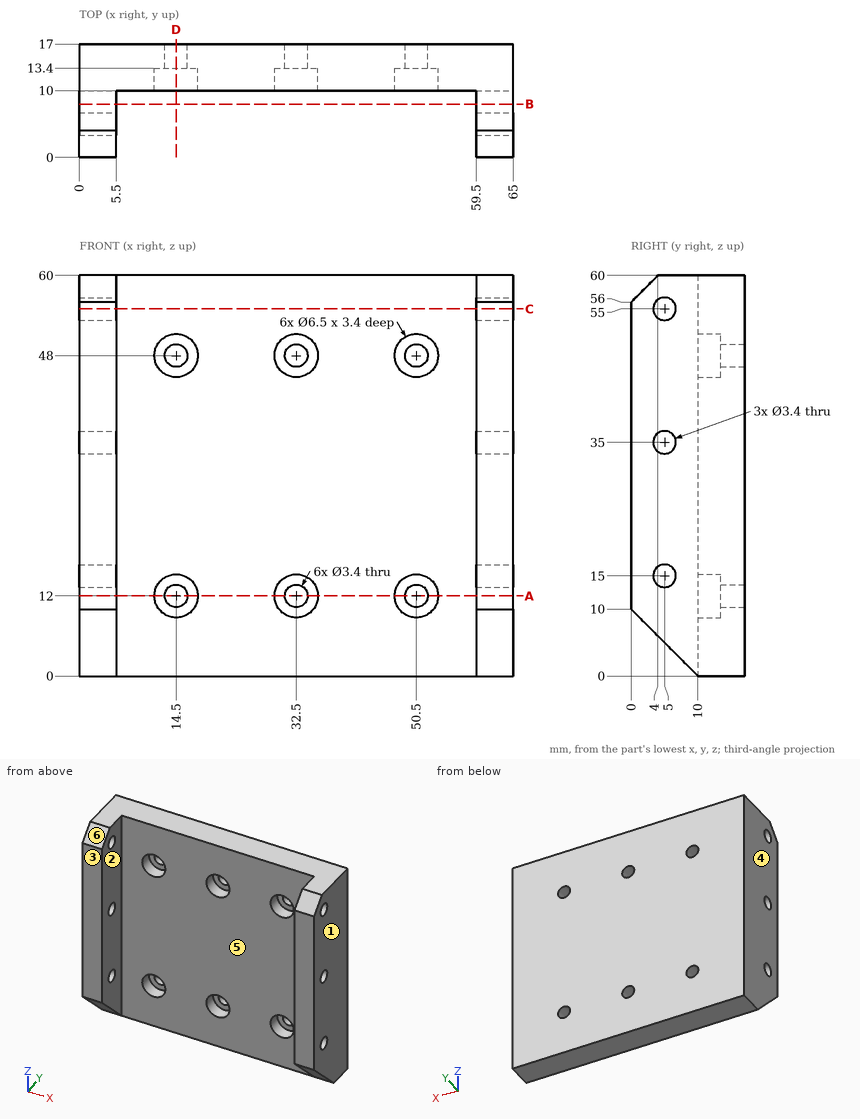
Geometry: see drawing. Coordinates: mm, zero at the bounding-box minimum. A direction names the side the tool comes from. Coordinates: 2 decimals unless noted, no trailing zeros. Loops run counter-clockwise (first coordinate to the right, second up) from the corner with the lowest first, then second, coordinate; pieces in that order, holes last. Notation, with made-up numbers: (-39.75, 62) -> (8.25, 62) arc R20 ccw to (8.25, 76) -> close; hole circle Ø8 at (15.5, -33). An arc over 180 degrees is marked (long way). Write item = value, one per line. Start each with the question number.
Item 1: Cut plane B-B, the plane y = 8. Return loops of the section in (x, z).
Item 2: Cut plane C-C, the plane z = 55. Return loops of the section in (x, y).
Item 3: Material intervals for line 1 (X direction, y = 15.35, z = 48); line 2 (Z direction, x = 14.5, y = 14.9); line 3 (X direction, y = 6, z = 49.5), sorted ascending.
Item 4: Reachability of the marked faces 5 and 6 from +Z, -Z, +X, -X, +Y, -Y: full face, straight path, thin tool, end or side. Return the list, or none.
Item 5: First-contact query: P1, Ø7, axis at x = 49, z = 49, coming from the -Y side; P2, Ø4, axis at x = 32.5, z = 12, coming from the -Y side. Flat tips, straight axial feed; report the tip coordinate or a pass-through.
Item 6: Mould query, pull axis X, two halves, no side actions, for the marked faces 1, 2, 3 and 4. Classes: pulls with the +X half, pulls with the -X half, needs draft (parallel to the pull), parting line crosses it, or undercut.
Item 7: Cut plane A-A, the plane z = 12. Count the separate pieces of the cut face and the enclosed holes in it, plus the area to 3 significant figures.
Item 8: Cut plane D-D, the plane x = 14.5. Return loops of the section in (y, z).
Ans:
q1.outline = (0, 2) -> (5.5, 2) -> (5.5, 60) -> (0, 60) -> close; (59.5, 2) -> (65, 2) -> (65, 60) -> (59.5, 60) -> close
q2.outline = (0, 0) -> (5.5, 0) -> (5.5, 3.3) -> (0, 3.3) -> close; (0, 6.7) -> (5.5, 6.7) -> (5.5, 10) -> (59.5, 10) -> (59.5, 6.7) -> (65, 6.7) -> (65, 17) -> (0, 17) -> close; (59.5, 0) -> (65, 0) -> (65, 3.3) -> (59.5, 3.3) -> close
q3.line_1 = 0 to 12.8, 16.2 to 30.8, 34.2 to 48.8, 52.2 to 65
q3.line_2 = 0 to 10.3, 13.7 to 46.3, 49.7 to 60
q3.line_3 = 0 to 5.5, 59.5 to 65
q4.face_5 = +Z, -Z, -Y
q4.face_6 = +Z, +X, -X, -Y
q5.P1 = 10
q5.P2 = 13.4
q6.face_1 = pulls with the +X half
q6.face_2 = undercut
q6.face_3 = needs draft
q6.face_4 = pulls with the -X half
q7.separate_pieces = 4
q7.enclosed_holes = 0
q7.area = 462 mm²
q8.outline = (10, 0) -> (17, 0) -> (17, 10.3) -> (13.4, 10.3) -> (13.4, 8.75) -> (10, 8.75) -> close; (10, 15.25) -> (13.4, 15.25) -> (13.4, 13.7) -> (17, 13.7) -> (17, 46.3) -> (13.4, 46.3) -> (13.4, 44.75) -> (10, 44.75) -> close; (10, 51.25) -> (13.4, 51.25) -> (13.4, 49.7) -> (17, 49.7) -> (17, 60) -> (10, 60) -> close
